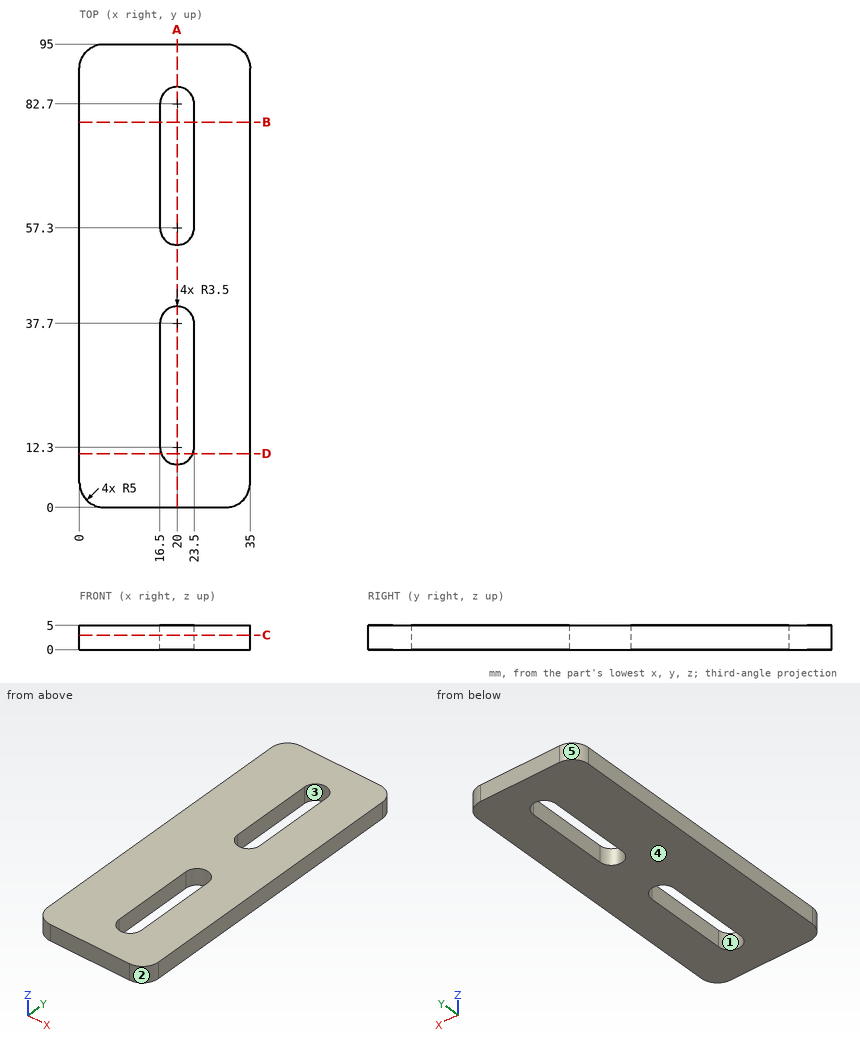
Input: dimensioned drawing with shaded views. Units: mm. Origin: part minimum x, y, z. A direction names the side the tool comes from. Coordinates: 2 decimals unless noted, no trailing zeros. Order: outer loops, then holes, each group sorted by start corner. A loop starts at its lowest first (then second) coordinate and runs counter-clockwise, first axis right, second up. Notation, with made-up numbers: (52.5, 48) -> (99.5, 48) arc R24 ccw to (99.5, 84) -> close; hole circle Ø2 at (60.5, 9). An arc over 180 degrees is marked (long way). Use CSV: the item, a comma, the result in double quotes.
1) Section B-B on y = 79. Output: boundary loops of the cut face in (x, z), then the cut area to 3 significant figures.
Findings:
outline,"(0, 0) -> (16.5, 0) -> (16.5, 5) -> (0, 5) -> close; (23.5, 0) -> (35, 0) -> (35, 5) -> (23.5, 5) -> close"
area,"140 mm^2"
2) Section C-C on z = 3. Output: boundary loops of the cut face in (x, y).
Findings:
outline,"(0, 5) arc R5 ccw to (5, 0) -> (30, 0) arc R5 ccw to (35, 5) -> (35, 90) arc R5 ccw to (30, 95) -> (5, 95) arc R5 ccw to (0, 90) -> close; hole (16.5, 12.3) arc R3.5 ccw to (23.5, 12.3) -> (23.5, 37.7) arc R3.5 ccw to (16.5, 37.7) -> close; hole (16.5, 57.3) arc R3.5 ccw to (23.5, 57.3) -> (23.5, 82.7) arc R3.5 ccw to (16.5, 82.7) -> close"
3) Mould query, pull axis Y, two halves, no side actions, for the marked faces 3, 4 and 5. Classes: +Y half, -Y half, draft (parallel to the pull), parting line (faces both ways), or undercut.
Findings:
face 3,"undercut"
face 4,"draft"
face 5,"+Y half"
4) Pin query (flat end, axial travel): pin 1 Ø1 at (x, z) = (24, 3) entering from -Y. Return the tip coordinate at first contact, or that it passes through.
Findings:
pin 1,"stops at y = 0"
5) Section A-A on x = 20. Output: boundary loops of the cut face in (y, z), then the cut area to 3 significant figures.
Findings:
outline,"(0, 0) -> (8.8, 0) -> (8.8, 5) -> (0, 5) -> close; (41.2, 0) -> (53.8, 0) -> (53.8, 5) -> (41.2, 5) -> close; (86.2, 0) -> (95, 0) -> (95, 5) -> (86.2, 5) -> close"
area,"151 mm^2"
6) Section D-D on y = 11. Output: boundary loops of the cut face in (x, z).
Findings:
outline,"(0, 0) -> (16.75, 0) -> (16.75, 5) -> (0, 5) -> close; (23.25, 0) -> (35, 0) -> (35, 5) -> (23.25, 5) -> close"
7) Line query: line 1 (X direction, y = 58, z = 4); line 2 (Y direction, x = 19.5, z = 2.1); line 3 (Y direction, x = 17, z = 3.2). Output: solid intervals per line, ascending.
Findings:
line 1,"x = 0 to 16.5, 23.5 to 35"
line 2,"y = 0 to 8.84, 41.16 to 53.84, 86.16 to 95"
line 3,"y = 0 to 10.5, 39.5 to 55.5, 84.5 to 95"
8) Access query for the marked faces 1 and 2. Directions: +Z, -Z, +X, -X, +Y, -Y. A direction counts if a zero-diameter tool reaches every point of the face in a straight line with its end or side. Return the directions, or none.
Findings:
face 1,"+Z, -Z"
face 2,"+Z, -Z, +X, -Y"
